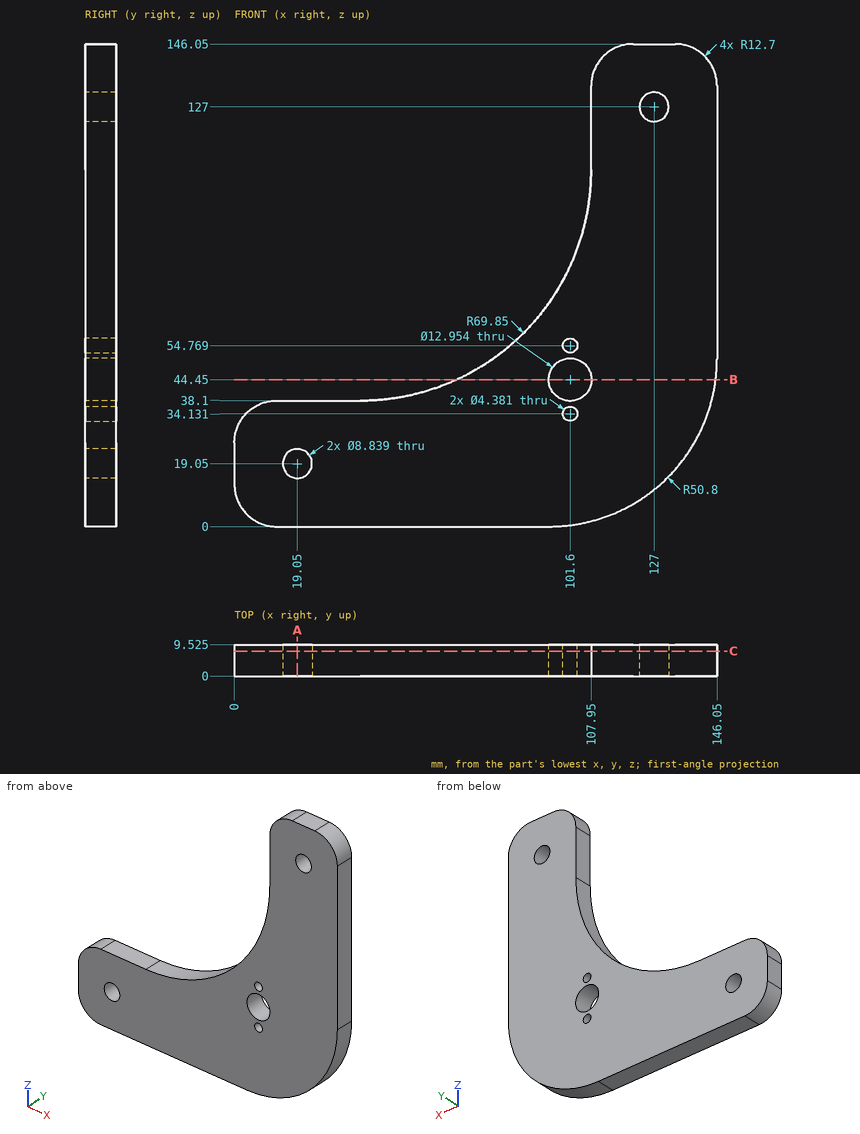
Study the drawing (mm; zero at the part's minimum x, y, z) and answer. Give positions to 0.01 mm unless a question says otherwise; leave off trailing zeros. Write each loop counter-clockwise with the first axis right and the second up, starting at its lowest first coordinate (ties: lowest second). Pieces come first, ordered by that corner, then holes. Notation, with made-up numbers: (40, 87.25) - (82, 87.25) arc R27 cw to (82, 106.25) - close; hole circle Ø4 at (85, 66). An arc over 180 degrees is marked (long way). Write item = value, one per line. Start each with the question number.
Item 1: Find the intervals of material crossed by probe 1 along X at (y, z) = (7.75, 106); probe 2 along X at (y, z) = (2.5, 129); probe 3 along Z at (x, y) = (31, 1.75), in increasing order. Write a range as [from, to].
Item 2: Find section A-A (x = 19.05). Give the vertices of the cut face in (y, z) (1 decimal).
Item 3: Each of these flat-tipped pins is pushed along its axis until it touches: P1, Ø1.5, axis at y = 7.5, z = 37, coming from the +X side (1 decimal); P2, Ø1.5, axis at y = 3.5, z = 129.5, coming from the -X side; P3, Ø8, axis at x = 19.05, z = 19.05, coming from the +Y side; P4, Ø5, axis at x = 26, y = 6.5, coming from the +Z side. Where does it stop, or does it pass through?
Item 4: Find section B-B (z = 44.45). Give the vertices of the cut face in (x, y) (1 decimal).
Item 5: Find section C-C (y = 7.5). State how many separate pieces and enclosed holes the cut face has, then the cut area to 3 significant figures.
Response:
q1.probe_1 = [107.92, 146.05]
q1.probe_2 = [107.95, 123.06], [130.94, 146.05]
q1.probe_3 = [0, 38.1]
q2.outline = (0, 0) - (9.5, 0) - (9.5, 14.6) - (0, 14.6) - close; (0, 23.5) - (9.5, 23.5) - (9.5, 38.1) - (0, 38.1) - close
q3.P1 = 144.3
q3.P2 = 107.95
q3.P3 = through
q3.P4 = 38.1
q4.outline = (67.2, 0) - (95.1, 0) - (95.1, 9.5) - (67.2, 9.5) - close; (108.1, 0) - (145.7, 0) - (145.7, 9.5) - (108.1, 9.5) - close
q5.separate_pieces = 1
q5.enclosed_holes = 5
q5.area = 9,750 mm²
